The drawing under review shows one solid part. Ordinate dimensions are in mm from its lowest x, y, z. A direction names the side the tool comes from. Round coordinates to 2 decimals unless told otherwise and drop trailing zeros. Write each loop counter-clockwise with the first axis right and the second up, starting at its lowest first coordinate (ties: lowest second). Pieces come first, ordered by that corner, then holes. Notation, with made-up numbers: M 10.25,85.5 L 40.25,85.5 A27 cw 40.25,118.5 Z; hole C 71,-30 d11. An arc over 180 degrees is marked long. One line per item, written item: value. Start each with the question number.
1) Wall thickness on probe 1 along Y at (x, z) = (5, 8.8); probe 2 along Y at (x, z) = (72, 6.7); probe 3 along Y at (x, z) = (14, 7.75): over which ranges is each line inside the solid? List them lowest first.
2) Take a section at D-D, the plane x = 5. Write out the cut boundary in (y, z), and give its area (3 significant figures).
3) For P1, Ø1.5, axis at x = 102, z = 5, coming from the -Y side; P2, Ø3, axis at y = 38.5, z = 8.5, coming from the +X side; P3, Ø4, axis at x = 6, z = 8, coming from the -Y side, all flat-tipped, find the tip position at first contact; note any pin that passes through.
4) Take a section at A-A, the plane y = 72. Write out the cut boundary in (x, z).
5) Tool access review of the marked faces 1, 2 and 3: name each direction out of +Z, -Z, +X, -X, +Y, -Y from which nothing blocks a thin tool from reaching the whole face with its end or side.
6) Take a section at B-B, the plane x = 72. Write out the cut boundary in (y, z), and give its area (4 significant figures).
7) Take a section at C-C, the plane z = 7.75. Write out the cut boundary in (x, y).
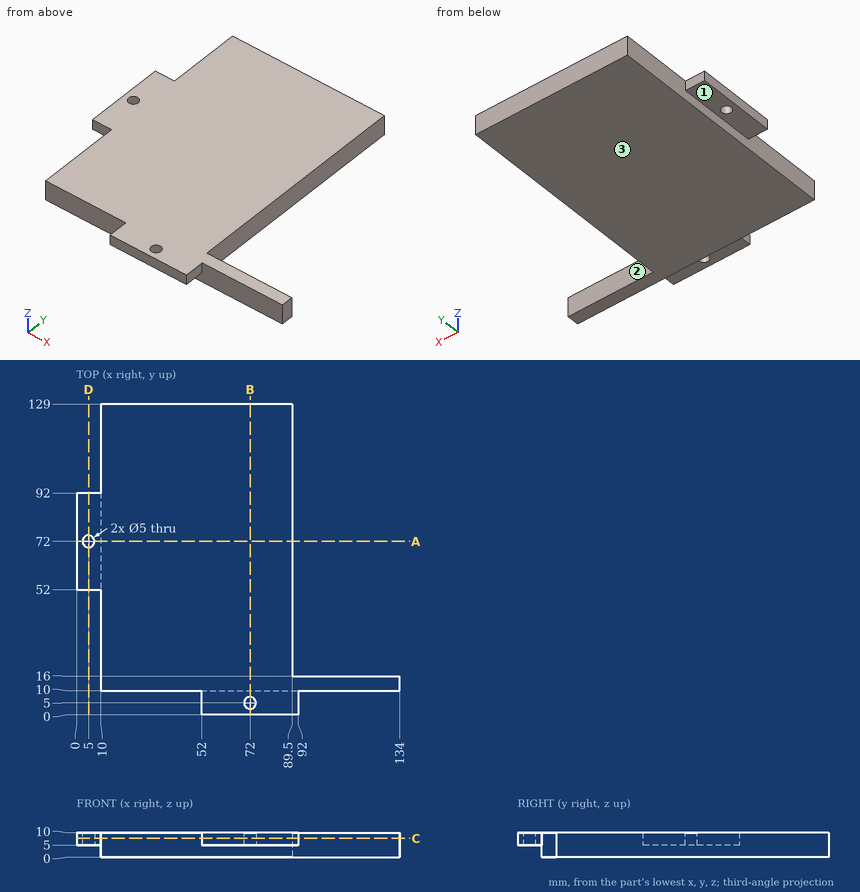
Checked values:
1. probe 1: y = 52 to 69.5, 74.5 to 92
1. probe 2: y = 0 to 2.5, 7.5 to 129
1. probe 3: y = 10 to 129
2. outline: M 52,5 L 69.5,5 L 69.5,10 L 52,10 Z; M 74.5,5 L 92,5 L 92,10 L 74.5,10 Z
2. area: 175 mm2
3. P1: stops at y = 10
3. P2: stops at x = 89.5
3. P3: stops at y = 52
4. outline: M 0,5 L 2.5,5 L 2.5,10 L 0,10 Z; M 7.5,5 L 10,5 L 10,0 L 89.5,0 L 89.5,10 L 7.5,10 Z
5. face 1: -Z, -X, +Y, -Y
5. face 2: +Z, -Z, +X, +Y
5. face 3: -Z, +X, -X, +Y, -Y
6. outline: M 0,5 L 2.5,5 L 2.5,10 L 0,10 Z; M 7.5,5 L 10,5 L 10,0 L 129,0 L 129,10 L 7.5,10 Z
6. area: 1,215 mm2
7. outline: M 0,52 L 10,52 L 10,10 L 52,10 L 52,0 L 92,0 L 92,10 L 134,10 L 134,16 L 89.5,16 L 89.5,129 L 10,129 L 10,92 L 0,92 Z; hole C 5,72 d5; hole C 72,5 d5
